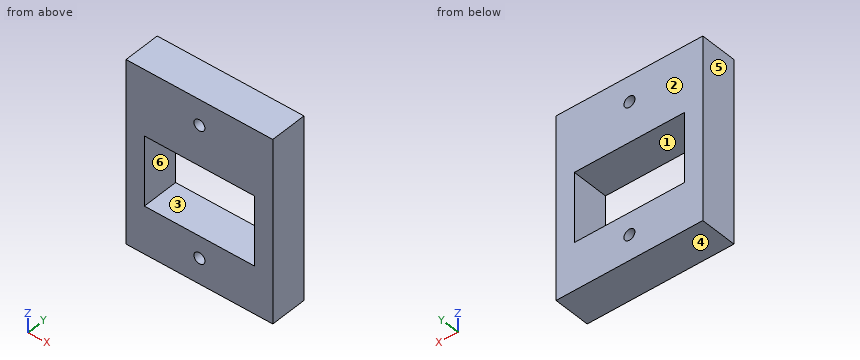
Autodesk Inventor part; units mm, degrees
ref_plane "YZ Plane" through (0, 0, 0) normal (1, 0, 0) x (0, 1, 0)
ref_plane "XZ Plane" through (0, 0, 0) normal (0, 1, 0) x (-1, 0, 0)
ref_plane "XY Plane" through (0, 0, 0) normal (0, 0, 1) x (1, 0, 0)
sketch "Sketch1" plane through (0, 0, 0) normal (0, 1, 0) x (-1, 0, 0)
  line L0 (0, 0) -> (40, 0)
  line L1 (40, 0) -> (40, -50)
  line L2 (40, -50) -> (0, -50)
  line L3 (0, -50) -> (0, 0)
  line L4 (40, 0) -> (0, 0)
  line L5 (0, 0) -> (0, -18)
  line L6 (5, -18) -> (35, -18)
  line L7 (40, -18) -> (40, 0)
  line L8 (35, -18) -> (5, -18)
  line L9 (0, -18) -> (0, -37)
  line L10 (5, -37) -> (35, -37)
  line L11 (40, -37) -> (40, -18)
  circle A0 centre (20, -7) radius 1.5
  circle A1 centre (20, -43) radius 1.5
  line L12 (20, -18) -> (35, -18)
  line L13 (35, -18) -> (35, -37)
  line L14 (35, -37) -> (20, -37)
  line L15 (20, -37) -> (5, -37)
  line L16 (5, -37) -> (5, -18)
  line L17 (5, -18) -> (20, -18)
  dimension "d0" = 40
  dimension "d1" = 50
  dimension "d2" = 3
  dimension "d3" = 3
extrude "Extrusion1" add sketch "Sketch1" along normal blind 10
properties part number "_3DPrint"
Verification items for the finished model (mm, model axes). Face numbers are marked on the shaded views. A direction names the side the tool comes from. Coordinates: 2 decimals unless noted, no trailing zeros. Order: outer loops, then holes, each group sorted by start corner. A loop starts at its lowest first (then second) coordinate and runs counter-clockwise, first axis right, second up.
Item 1: Section check D-D, the plane y = 5.25. Enter the section's corners in (x, z), then the cut area to 3 significant figures.
Filled in:
outline: (-40, -50) - (0, -50) - (0, 0) - (-40, 0) - close; hole (-35, -37) - (-5, -37) - (-5, -18) - (-35, -18) - close; hole circle Ø3 at (-20, -43); hole circle Ø3 at (-20, -7)
area: 1,420 mm2
Item 2: Section check C-C, the plane x = -25. Enter the section's corners in (y, z), then the cut area to 3 significant figures.
Filled in:
outline: (0, -50) - (10, -50) - (10, -37) - (0, -37) - close; (0, -18) - (10, -18) - (10, 0) - (0, 0) - close
area: 310 mm2
Item 3: Access from +Z, -Z, +X, -X, +Y, -Y to the whole of each face (thin tool, end or side, straight path). Record for the marked faces 5 and 6.
Filled in:
face 5: +Z, -Z, -X, +Y, -Y
face 6: +Y, -Y
Item 4: Material ranges on L1, parallel to Z at x = -20, y = 7; L2, parallel to X at y = 4, z = -31; L3, parallel to Z at x = -6.5, y = 4.5, recorded low to high.
Filled in:
L1: z = -50 to -44.5, -41.5 to -37, -18 to -8.5, -5.5 to 0
L2: x = -40 to -35, -5 to 0
L3: z = -50 to -37, -18 to 0
Item 5: Section check B-B, the plane x = -20. Enter the section's corners in (y, z), then the cut area to 3 significant figures.
Filled in:
outline: (0, -50) - (10, -50) - (10, -44.5) - (0, -44.5) - close; (0, -41.5) - (10, -41.5) - (10, -37) - (0, -37) - close; (0, -18) - (10, -18) - (10, -8.5) - (0, -8.5) - close; (0, -5.5) - (10, -5.5) - (10, 0) - (0, 0) - close
area: 250 mm2
Item 6: Release check for a two-part mould opening along Z. For the marked faces 1, 2, 3 and 4 record: +Z half, -Z half, draft (parallel to the pull), parting line (faces both ways), or undercut.
Filled in:
face 1: undercut
face 2: draft
face 3: undercut
face 4: -Z half
Item 7: Section check A-A, the plane z = -21.5. Enter the section's corners in (x, y), then the cut area to 3 significant figures.
Filled in:
outline: (-40, 0) - (-35, 0) - (-35, 10) - (-40, 10) - close; (-5, 0) - (0, 0) - (0, 10) - (-5, 10) - close
area: 100 mm2
